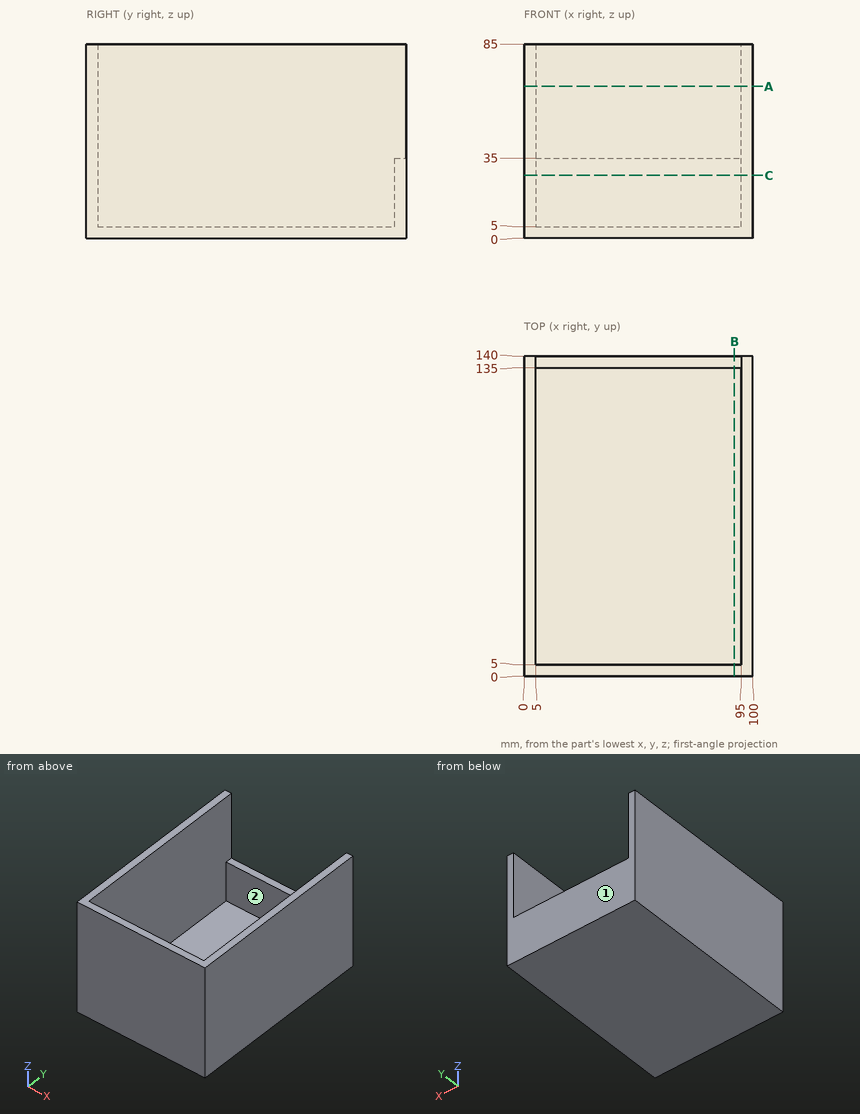
Verification items for this drawing (mm, ordinates from the low corner). A direction names the side the tool comes from. Round coordinates to 2 decimals unless told otherwise and drop trailing zeros. Order: outer loops, then holes, each group sorted by start corner. A loop starts at its lowest first (then second) coordinate and runs counter-clockwise, first axis right, second up. Notation, with made-up numbers: (42.5, 28.5) - (54.5, 28.5) arc R20 ccw to (54.5, 34.5) - close; hole circle Ø3 at (-5.75, 1). An arc over 180 degrees is marked (long way). Use CSV: the item, a comma, the result in double quotes. Start each with the question number.
1) Go/stop test with flat-tipped pins: P1, Ø2.5, axis at x = 45.5, y = 138, coming from the +Z side; P2, Ø4, axis at x = 22, y = 37, coming from the +Z side. Record where each tip stops, or that it passes through.
2) Section check B-B, the plane x = 92. Record the cut outline in (y, z), plus the area to 3 significant figures.
3) Thickness scan on L1, parallel to X at y = 99.5, z = 47; L2, parallel to Y at x = 49, z = 32.5; L3, parallel to Y at x = 31, z = 65.5. Record the ranges inside material, lowest first.
4) Access from +Z, -Z, +X, -X, +Y, -Y to the whole of each face (thin tool, end or side, straight path). Record for the marked faces 1 and 2.
5) Section check A-A, the plane z = 66.5. Record the cut outline in (x, y).
6) Section check C-C, the plane z = 27.5. Record the cut outline in (x, y).
Answers:
1,P1,"stops at z = 35"
1,P2,"stops at z = 5"
2,outline,"(0, 0) - (140, 0) - (140, 35) - (135, 35) - (135, 5) - (5, 5) - (5, 85) - (0, 85) - close"
2,area,"1,250 mm²"
3,L1,"x = 0 to 5, 95 to 100"
3,L2,"y = 0 to 5, 135 to 140"
3,L3,"y = 0 to 5"
4,face 1,"+Z, -Z, +X, -X, +Y"
4,face 2,"+Z"
5,outline,"(0, 0) - (100, 0) - (100, 140) - (95, 140) - (95, 5) - (5, 5) - (5, 140) - (0, 140) - close"
6,outline,"(0, 0) - (100, 0) - (100, 140) - (0, 140) - close; hole (5, 5) - (95, 5) - (95, 135) - (5, 135) - close"
